Verification items for the finished model (mm, model axes). Round coordinates to 2 decimals unless told otherwise and drop trailing zeros. Write each loop counter-clockwise with the first axis right and the second up, starting at its lowest first coordinate (ties: lowest second). Pieces come first, ordered by that corner, then holes. Notation, with made-up numbers: M 29,-33.5 L 58,-33.5 A18 cw 58,-17.5 Z; hole C -39,-37 d7. An arc over 180 degrees is marked long. One line per question, with ' | ' between items. Start each with the question number.
Q1. Thickness scan on line 1 along X through (y, z) = (2.35, 13.5); line 2 along X through (y, z) = (2.3, -14); line 3 along Z through (x, y) = (-39, 3.65). Record the ranges inside material, lowest first. Write a range as from..to.
Q2. Cross-section at C-C (y = 2.7). State how many separate pieces and enclosed holes the cut face has, then the cut area to 3 significant figures.
Q3. Cross-section at B-B (x = -28). Record the boundary of the cut face in (y, z), then the cut area to 3 significant figures.
Q4. Cross-section at A-A (z = 53.25). Record the boundary of the cut face in (x, y).
Q5. Gauge pin test, flat ends, axial feed: pin 1 (1.9 mm diameter, centred on x = 48.3, z = -15.01, fed in from -Y); pin 2 (2 mm diameter, centred on x = 6.5, y = 4, fed in from -Z); pin 3 (2 mm diameter, centred on y = 3.5, z = 23, fed in from +X); pin 4 (1.5 mm diameter, centred on x = 29.5, y = 2, fed in from -Z). Record the tip position at first contact, or that the pin passes through.
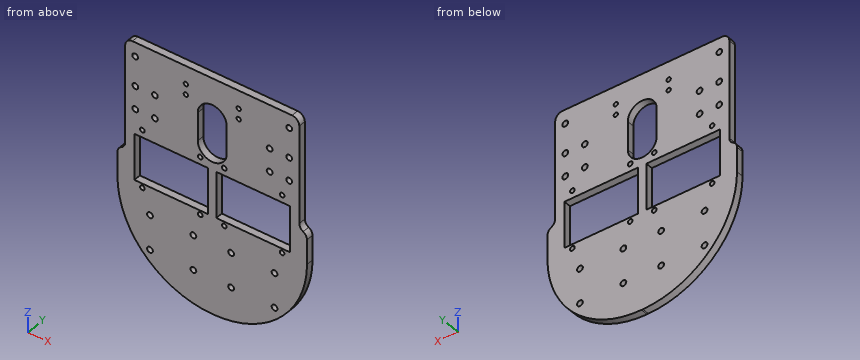
from build123d import *

# Parameters (mm, degrees)
BOSS_EXTRUDE2_DEPTH = 5
FILLET8_R           = 65
SKETCH4_R           = 2
SKETCH4_R_2         = 1.605
SKETCH4_R_3         = 1.5
SKETCH4_W           = 51
SKETCH4_H           = 32
CUT_EXTRUDE1_DEPTH  = 5
FILLET9_R           = 5
FILLET10_R          = 5


with BuildPart() as part:
    # Sketch1 → Boss-Extrude2 (new body)
    with BuildSketch(Plane(origin=(0, 0, 0), x_dir=(1, 0, 0), z_dir=(0, 1, 0))):
        Polygon((65.5, 80), (-65.5, 80), (-65.5, -7), (-60.15, -7), (-60.15, -83.5), (60.15, -83.5), (60.15, -7), (65.5, -7), align=None)
    extrude(amount=BOSS_EXTRUDE2_DEPTH)

    # Fillet8
    fillet8_edges = [part.edges().sort_by_distance(p)[0] for p in [
        (-65.5, 2.5, -80),
        (65.5, 2.5, -80),
    ]]
    fillet(fillet8_edges, radius=FILLET8_R)

    # Sketch4 → Cut-Extrude1 (cut)
    with BuildSketch(Plane(origin=(0, 5, 0), x_dir=(1, 0, 0), z_dir=(0, 1, 0))):
        with Locations(Location((-39.65, -37.25, 0), (0, 0, 270))):
            Circle(SKETCH4_R)
        with Locations(Location((39.65, -37.25, 0), (0, 0, 90))):
            Circle(SKETCH4_R)
        with Locations(Location((39.65, -53.25, 0), (0, 0, 270))):
            Circle(SKETCH4_R)
        with Locations(Location((-39.65, -53.25, 0), (0, 0, 90))):
            Circle(SKETCH4_R)
        with Locations(Location((-53.15, -37.25, 0), (0, 0, 270))):
            Circle(SKETCH4_R)
        with Locations(Location((-53.15, -53.25, 0), (0, 0, 90))):
            Circle(SKETCH4_R)
        with Locations(Location((53.15, -53.25, 0), (0, 0, 270))):
            Circle(SKETCH4_R)
        with Locations(Location((53.15, -37.25, 0), (0, 0, 90))):
            Circle(SKETCH4_R)
        with Locations(Location((-48.298883815, 15.012633239, 0), (0, 0, 270))):
            Circle(SKETCH4_R_2)
        with Locations(Location((-8.298883815, 15.012633239, 0), (0, 0, 270))):
            Circle(SKETCH4_R_2)
        with Locations(Location((-48.298883815, -24.987366761, 0), (0, 0, 270))):
            Circle(SKETCH4_R_2)
        with Locations(Location((-8.298883815, -24.987366761, 0), (0, 0, 270))):
            Circle(SKETCH4_R_2)
        with Locations(Location((48.298883815, -24.987366761, 0), (0, 0, 90))):
            Circle(SKETCH4_R_2)
        with Locations(Location((8.298883815, -24.987366761, 0), (0, 0, 90))):
            Circle(SKETCH4_R_2)
        with Locations(Location((8.298883815, 15.012633239, 0), (0, 0, 90))):
            Circle(SKETCH4_R_2)
        with Locations(Location((48.298883815, 15.012633239, 0), (0, 0, 90))):
            Circle(SKETCH4_R_2)
        with Locations(Location((13.047144734, 55.54428083, 0), (0, 0, 270))):
            Circle(SKETCH4_R)
        with Locations(Location((43.047144734, 55.54428083, 0), (0, 0, 270))):
            Circle(SKETCH4_R)
        with Locations(Location((43.047144734, 31.54428083, 0), (0, 0, 270))):
            Circle(SKETCH4_R)
        with Locations(Location((13.047144734, 31.54428083, 0), (0, 0, 270))):
            Circle(SKETCH4_R)
        with Locations(Location((-43.047144734, 55.54428083, 0), (0, 0, 90))):
            Circle(SKETCH4_R)
        with Locations(Location((-43.047144734, 31.54428083, 0), (0, 0, 90))):
            Circle(SKETCH4_R)
        with Locations(Location((-13.047144734, 31.54428083, 0), (0, 0, 90))):
            Circle(SKETCH4_R)
        with Locations(Location((-13.047144734, 55.54428083, 0), (0, 0, 90))):
            Circle(SKETCH4_R)
        with Locations(Location((-18.248740478, -71, 0), (0, 0, 270))):
            Circle(SKETCH4_R_3)
        with Locations(Location((-53.249046458, -73.796312774, 0), (0, 0, 270))):
            Circle(SKETCH4_R)
        with Locations(Location((53.249046458, -73.796312774, 0), (0, 0, 90))):
            Circle(SKETCH4_R)
        with Locations(Location((18.251259522, -71, 0), (0, 0, 270))):
            Circle(SKETCH4_R_3)
        with Locations(Location((-18.248740478, -63.7, 0), (0, 0, 270))):
            Circle(SKETCH4_R_3)
        with Locations(Location((18.25125952, -63.7, 0), (0, 0, 270))):
            Circle(SKETCH4_R_3)
        with BuildLine():
            Line((10, -35.5), (10, -55))
            ThreePointArc((10, -55), (0, -65), (-10, -55))
            Line((-10, -55), (-10, -35.5))
            ThreePointArc((-10, -35.5), (0, -25.5), (10, -35.5))
        make_face()
        with Locations((-28.298883815, -3.887366761)):
            Rectangle(SKETCH4_W, SKETCH4_H)
        with Locations((28.298883815, -3.887366761)):
            Rectangle(SKETCH4_W, SKETCH4_H)
    extrude(amount=-CUT_EXTRUDE1_DEPTH, mode=Mode.SUBTRACT)

    # Fillet9
    fillet9_edges = [part.edges().sort_by_distance(p)[0] for p in [
        (60.15, 2.5, 83.5),
        (-60.15, 2.5, 83.5),
        (-65.5, 2.5, 7),
        (65.5, 2.5, 7),
    ]]
    fillet(fillet9_edges, radius=FILLET9_R)

    # Fillet10
    fillet10_edges = [part.edges().sort_by_distance(p)[0] for p in [
        (60.15, 2.5, 7),
        (-60.15, 2.5, 7),
    ]]
    fillet(fillet10_edges, radius=FILLET10_R)


solid = part.part
Determined:
1) line 1: x = -60.15..-53.8, -2.8..2.8, 53.8..60.15 | line 2: x = -65.5..-49.54, -47.05..-9.54, -7.05..7.05, 9.54..47.05, 49.54..65.5 | line 3: z = -67.37..-12.11, 19.89..35.36, 39.14..51.36, 55.14..83.5
2) separate pieces: 1 | enclosed holes: 33 | area: 14,500 mm²
3) outline: M 0,-73.9 L 5,-73.9 L 5,-12.11 L 0,-12.11 Z; M 0,19.89 L 5,19.89 L 5,83.5 L 0,83.5 Z | area: 627 mm²
4) outline: M -60.15,0 L -55.15,0 L -55.15,5 L -60.15,5 Z; M -51.15,0 L -41.65,0 L -41.65,5 L -51.15,5 Z; M -37.65,0 L -10,0 L -10,5 L -37.65,5 Z; M 10,0 L 37.65,0 L 37.65,5 L 10,5 Z; M 41.65,0 L 51.15,0 L 51.15,5 L 41.65,5 Z; M 55.15,0 L 60.15,0 L 60.15,5 L 55.15,5 Z
5) pin 1: passes through | pin 2: stops at z = -79.81 | pin 3: stops at x = 60.15 | pin 4: stops at z = -73.54
